Model file for the job. Use its own axes, mm. A direction names the side the tool comes from. Round coordinates to 2 decimals unless told otherwise and drop trailing zeros. Loops run counter-clockwise (first coordinate to the right, second up) from the corner with the lowest first, then second, coordinate; pieces in that order, holes last. Notation, with made-up numbers: (-19.5, 31) -> (-10.5, 31) arc R26 ccw to (-10.5, 47) -> close; hole circle Ø1 at (39.5, -15). An arc over 180 degrees is marked (long way). Use a Markdown table: item, result. Add a question column.
```python
from build123d import *

# Parameters (mm, degrees)
BOSS_EXTRUDE1_DEPTH = 6.35
SKETCH2_W           = 18
SKETCH2_H           = 3
SKETCH2_W_2         = 10
SKETCH2_H_2         = 5
CUT_EXTRUDE1_DEPTH  = 148.509567486
SKETCH4_R           = 57.5
CUT_EXTRUDE2_DEPTH  = 148.509567486
SKETCH5_R           = 1.6
CUT_EXTRUDE3_DEPTH  = 148.509567486


with BuildPart() as part:
    # Sketch1 → Boss-Extrude1 (new body)
    with BuildSketch(Plane(origin=(0, 0, 0), x_dir=(1, 0, 0), z_dir=(0, 1, 0))):
        Polygon((64.951905284, 87.5), (-64.951905284, 87.5), (-108.253175473, 12.5), (-43.301270189, -100), (43.301270189, -100), (108.253175473, 12.5), align=None)
    extrude(amount=BOSS_EXTRUDE1_DEPTH)

    # Sketch2 → Cut-Extrude1 (cut, through all)
    with BuildSketch(Plane(origin=(0, 6.35, 0), x_dir=(1, 0, 0), z_dir=(0, 1, 0))):
        with Locations((-29, -92.2)):
            Rectangle(SKETCH2_W, SKETCH2_H)
        with Locations((29, -92.2)):
            Rectangle(SKETCH2_W, SKETCH2_H)
        Polygon((-62.146580335, 79.758965344), (-59.548504123, 78.258965344), (-68.548504123, 62.670508076), (-71.146580335, 64.170508076), align=None)
        Polygon((-97.548504123, 12.441034656), (-88.548504123, 28.029491924), (-91.146580335, 29.529491924), (-100.146580335, 13.941034656), align=None)
        Polygon((100.146580335, 13.941034656), (91.146580335, 29.529491924), (88.548504123, 28.029491924), (97.548504123, 12.441034656), align=None)
        Polygon((59.548504123, 78.258965344), (62.146580335, 79.758965344), (71.146580335, 64.170508076), (68.548504123, 62.670508076), align=None)
        with Locations((-29, -69.2)):
            Rectangle(SKETCH2_W_2, SKETCH2_H_2)
        with Locations((29, -69.2)):
            Rectangle(SKETCH2_W_2, SKETCH2_H_2)
        Polygon((79.094021451, 6.405136271), (74.094021451, 15.065390309), (69.763894432, 12.565390309), (74.763894432, 3.905136271), align=None)
        Polygon((40.763894432, 62.794863729), (45.094021451, 65.294863729), (50.094021451, 56.634609691), (45.763894432, 54.134609691), align=None)
        Polygon((-74.763894432, 3.905136271), (-69.763894432, 12.565390309), (-74.094021451, 15.065390309), (-79.094021451, 6.405136271), align=None)
        Polygon((-45.094021451, 65.294863729), (-40.763894432, 62.794863729), (-45.763894432, 54.134609691), (-50.094021451, 56.634609691), align=None)
    extrude(amount=-CUT_EXTRUDE1_DEPTH, mode=Mode.SUBTRACT)

    # Sketch4 → Cut-Extrude2 (cut, through all)
    with BuildSketch(Plane(origin=(0, 6.35, 0), x_dir=(1, 0, 0), z_dir=(0, 1, 0))):
        with Locations(Location((0, 0, 0), (0, 0, 270))):
            Circle(SKETCH4_R)
    extrude(amount=-CUT_EXTRUDE2_DEPTH, mode=Mode.SUBTRACT)

    # Sketch5 → Cut-Extrude3 (cut, through all)
    with BuildSketch(Plane(origin=(0, 6.35, 0), x_dir=(1, 0, 0), z_dir=(0, 1, 0))):
        with Locations(Location((0, 72.5, 0), (0, 0, 270))):
            Circle(SKETCH5_R)
        with Locations(Location((-62.786841774, -36.25, 0), (0, 0, 270))):
            Circle(SKETCH5_R)
        with Locations(Location((62.786841774, -36.25, 0), (0, 0, 270))):
            Circle(SKETCH5_R)
    extrude(amount=-CUT_EXTRUDE3_DEPTH, mode=Mode.SUBTRACT)


solid = part.part
```
1) Pin check, flat tips, straight feed: pin 1 Ø12 at (x, z) = (-37.5, -53) entering from -Y; pin 2 Ø1.5 at (y, z) = (4.5, 22) entering from +X; pin 3 Ø2.5 at (y, z) = (2.5, 92.5) entering from +X; pin 4 Ø3.5 at (y, z) = (3, 92) entering from -X. Stop position of each tip, or through.
2) Cut at A-A on x = -27. Write the cut outline in (y, z), and give its area (3 significant figures).
3) Cut at B-B on z = 0. Write the cut outline in (x, y), and give its area (3 significant figures).
4) Wall check: probe 1 along Z at (x, y) = (-61.5, 6); probe 2 along X at (y, z) = (4.5, 36.25); probe 3 along X at (y, z) = (1.5, 35). Give the ranges that are in metal, low to high. Write a range as from..to.
5) Pull direction X, two halves, no side cores. Call faces 3 (the face through (75.32, 3.13, 44.54)), 4 (the face through (-2, 6.35, -58)), 5 (the face through (29, 3, 66.7)): +X half, -X half, draft (parallel to the pull), parting line (faces both ways), or undercut.
6) Cut at D-D on y = 1.75. Count the separate pieces of the cut face and the enclosed holes in it, and give its area (3 significant figures).
7) Tool access for faces 1 (the face through (-76.232, 3.131, 42.963)), 2 (the face through (-72.3, 3.22, -8.17)): list every direction of +Z, -Z, +X, -X, +Y, -Y with a clear straight run to the whole face (end or side of a thin tool).
8) Cut at C-C on z = -22. Write the cut outline in (x, y), and give its area (3 significant figures).
Established:
| question | item | result |
|---|---|---|
| 1 | pin 1 | stops at y = 0 |
| 1 | pin 2 | stops at x = 88.77 |
| 1 | pin 3 | stops at x = 48.35 |
| 1 | pin 4 | stops at x = -48.93 |
| 2 | outline | (0, -87.5) -> (6.35, -87.5) -> (6.35, -50.77) -> (0, -50.77) -> close; (0, 50.77) -> (6.35, 50.77) -> (6.35, 66.7) -> (0, 66.7) -> close; (0, 71.7) -> (6.35, 71.7) -> (6.35, 90.7) -> (0, 90.7) -> close; (0, 93.7) -> (6.35, 93.7) -> (6.35, 100) -> (0, 100) -> close |
| 2 | area | 495 mm^2 |
| 3 | outline | (-101.04, 0) -> (-57.5, 0) -> (-57.5, 6.35) -> (-101.04, 6.35) -> close; (57.5, 0) -> (101.04, 0) -> (101.04, 6.35) -> (57.5, 6.35) -> close |
| 3 | area | 553 mm^2 |
| 4 | probe 1 | z = -87.5..-79.39, -74.88..35.3, 37.2..68.48 |
| 4 | probe 2 | x = -80.11..-64.39, -61.19..-44.63, 44.63..61.19, 64.39..80.11 |
| 4 | probe 3 | x = -80.83..-63.79, -61.79..-45.62, 45.62..61.79, 63.79..80.83 |
| 5 | face 3 | +X half |
| 5 | face 4 | draft |
| 5 | face 5 | undercut |
| 6 | separate pieces | 1 |
| 6 | enclosed holes | 16 |
| 6 | area | 19,000 mm^2 |
| 7 | face 1 | +Z, -X, +Y, -Y |
| 7 | face 2 | +Y, -Y |
| 8 | outline | (-102.77, 0) -> (-95.49, 0) -> (-95.49, 6.35) -> (-102.77, 6.35) -> close; (-92.03, 0) -> (-53.12, 0) -> (-53.12, 6.35) -> (-92.03, 6.35) -> close; (53.12, 0) -> (92.03, 0) -> (92.03, 6.35) -> (53.12, 6.35) -> close; (95.49, 0) -> (102.77, 0) -> (102.77, 6.35) -> (95.49, 6.35) -> close |
| 8 | area | 586 mm^2 |
